Verification items for the finished model (mm, model axes). Face numbers are marked on the shaded views. A direction names the side the tool comes from. Coordinates: 2 decimals unless noted, no trailing zeros. Write each loop counter-clockwise with the first axis right and the second up, starting at its lowest first coordinate (ties: lowest second). Pieces come first, ordered by that corner, then holes.
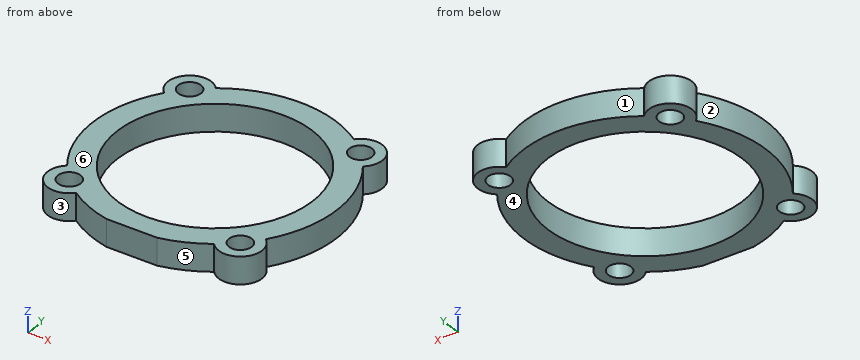
```python
from build123d import *

# Parameters (mm, degrees)
F1_DEPTH = 5
F2_R     = 2.1
F3_DEPTH = 5.001
F4_R     = 18
F5_DEPTH = 5.001


with BuildPart() as f1:
    # F0 (on Top) → F1 (new body)
    with BuildSketch(Plane.XY):
        with BuildLine():
            ThreePointArc((18.475718, 12.841256), (18.73833, 18.73833), (12.841256, 18.475718))
            ThreePointArc((12.841256, 18.475718), (0, 22.5), (-12.841256, 18.475718))
            ThreePointArc((-12.841256, 18.475718), (-18.73833, 18.73833), (-18.475718, 12.841256))
            ThreePointArc((-18.475718, 12.841256), (-22.5, 0), (-18.475718, -12.841256))
            ThreePointArc((-18.475718, -12.841256), (-18.73833, -18.73833), (-12.841256, -18.475718))
            ThreePointArc((-12.841256, -18.475718), (-8.954225, -20.641508), (-4.716991, -22))
            Line((-4.716991, -22), (4.716991, -22))
            ThreePointArc((4.716991, -22), (8.954225, -20.641508), (12.841256, -18.475718))
            ThreePointArc((12.841256, -18.475718), (18.73833, -18.73833), (18.475718, -12.841256))
            ThreePointArc((18.475718, -12.841256), (22.5, 0), (18.475718, 12.841256))
        make_face()
    extrude(amount=F1_DEPTH)

    # F2 (on face) → F3 (cut, through all)
    with BuildSketch(Plane.XY.offset(5)):
        with Locations((-15.909903, 15.909903)):
            Circle(F2_R)
        with Locations((15.909903, 15.909903)):
            Circle(F2_R)
        with Locations((15.909903, -15.909903)):
            Circle(F2_R)
        with Locations((-15.909903, -15.909903)):
            Circle(F2_R)
    extrude(amount=-F3_DEPTH, mode=Mode.SUBTRACT)

    # F4 (on face) → F5 (cut, through all)
    with BuildSketch(Plane.XY.offset(5)):
        Circle(F4_R)
    extrude(amount=-F5_DEPTH, mode=Mode.SUBTRACT)


solid = f1.part
```
1. Sectioned sample at D-D, the plane z = 3.3. Record the boundary of the cut face in (x, y), and give its area (3 significant figures).
2. Gauge pin test, flat ends, axial feed: P1, Ø2.5, axis at x = 15.91, y = 15.91, coming from the +Z side; P2, Ø1.5, axis at y = 16.5, z = 1, coming from the +X side; P3, Ø3, axis at y = 16, z = 4.5, coming from the -X side. Record the tip position at first contact, or that the pin passes through.
3. Sectioned sample at A-A, the plane y = 0. Record the boundary of the cut face in (x, z), and give its area (3 significant figures).
4. Draft check along Y on the marked faces 1, 2, 3 and 4. Enter one of: pulls with the +Y half, pulls with the -Y half, needs draft (parallel to the pull), parting line crosses it, or undercut.
5. Sectioned sample at B-B, the plane x = 0. Record the boundary of the cut face in (y, z).
6. Sectioned sample at C-C, the plane x = -15. Record the boundary of the cut face in (y, z), and give its area (3 significant figures).
7. Tool access check on the marked faces 5 and 6. Record the directions out of +Z, -Z, +X, -X, +Y, -Y that give a thin tool (end or side, any length) a straight path to the whole face; none if there is none.
8. Material ranges on L1, parallel to Y at x = 0, z = 3.15; L2, parallel to Y at x = -19.5, z = 3.75; L3, parallel to Y at x = -15.5, z = 4.6, recorded low to high.
Outcome:
1. outline: (-18.48, -12.84) arc R4 ccw (long way) to (-12.84, -18.48) arc R22.5 ccw to (-4.72, -22) - (4.72, -22) arc R22.5 ccw to (12.84, -18.48) arc R4 ccw (long way) to (18.48, -12.84) arc R22.5 ccw to (18.48, 12.84) arc R4 ccw (long way) to (12.84, 18.48) arc R22.5 ccw to (-12.84, 18.48) arc R4 ccw (long way) to (-18.48, 12.84) arc R22.5 ccw to start; hole circle Ø4.2 at (-15.91, -15.91); hole circle Ø4.2 at (-15.91, 15.91); hole circle Ø36 at (0, 0); hole circle Ø4.2 at (15.91, -15.91); hole circle Ø4.2 at (15.91, 15.91)
1. area: 618 mm2
2. P1: passes through
2. P2: stops at x = 19.91
2. P3: stops at x = -19.91
3. outline: (-22.5, 0) - (-18, 0) - (-18, 5) - (-22.5, 5) - close; (18, 0) - (22.5, 0) - (22.5, 5) - (18, 5) - close
3. area: 45.0 mm2
4. face 1: pulls with the +Y half
4. face 2: undercut
4. face 3: undercut
4. face 4: needs draft
5. outline: (-22, 0) - (-18, 0) - (-18, 5) - (-22, 5) - close; (18, 0) - (22.5, 0) - (22.5, 5) - (18, 5) - close
6. outline: (-19.81, 0) - (-17.8, 0) - (-17.8, 5) - (-19.81, 5) - close; (-14.02, 0) - (-9.95, 0) - (-9.95, 5) - (-14.02, 5) - close; (9.95, 0) - (14.02, 0) - (14.02, 5) - (9.95, 5) - close; (17.8, 0) - (19.81, 0) - (19.81, 5) - (17.8, 5) - close
6. area: 60.7 mm2
7. face 5: +Z, -Z, -Y
7. face 6: +Z, +X, -X, +Y, -Y
8. L1: y = -22 to -18, 18 to 22.5
8. L2: y = -17.67 to -14.15, -11.22 to 11.22, 14.15 to 17.67
8. L3: y = -19.89 to -17.97, -13.85 to -9.15, 9.15 to 13.85, 17.97 to 19.89
